Here's the drawing with two shaded views (mm, measured from the low corner). I have some questions. A direction names the side the tool comes from. Give positions to 0.01 mm unless a question says otherwise; leave off trailing zeros. Loops run counter-clockwise (first coordinate to the right, second up) from the corner with the lowest first, then second, coordinate; pieces in that order, holes last. Notation, with made-up numbers: (-12.75, 24.5) -> (-3.75, 24.5) arc R22 cw to (-3.75, 61.5) -> close; hole circle Ø10 at (-13.75, -13). An arc over 180 degrees is marked (long way). Answer in a Markdown table with one row per item. Add a question column.
Item 1: If I drill on line 1 (Y direction, x = 5.75, z = 14.5); line 2 (X direction, y = 59, z = 23); line 3 (Z direction, x = 32, y = 29.5), over which ranges is the centre line in solid material (lowest first)?
Item 2: If we section it at C-C (x = 5.75): Write out the boundary of the cut face in (y, z).
Item 3: If we section it at A-A (z = 11): Write out the boundary of the cut face in (x, y).
Item 4: Which directions (+Z, -Z, +X, -X, +Y, -Y) give clear straight access to the entire face, cutting with the end or side of a thin tool? Please do the marked faces 4, 5 and 6.
Item 5: For P1, Ø16, axis at x = 10, y = 45.5, coming from the -Z side; P2, Ø6.5, axis at x = 5.75, y = 60, coming from the +Z side; P3, Ø10, axis at x = 27, y = 46.5, coming from the -Z side; P4, Ø4.5, axis at x = 31.5, y = 18, coming from the -Z side, each with a flat end and sliding along its axis, tell me the tip position at first contact or that it passes through.
Item 6: If we section it at B-B (y = 10): Write out the boundary of the cut face in (x, z), then the cut area to 3 significant figures.
Item 7: We'd pull the mould along Z, two halves only. Please class the marked faces 1, 2 and 3: released by +Z, released by -Z, zero draft, split by the parting line, or undercut.
Item 8: If we section it at D-D (y = 63): Write out the boundary of the cut face in (x, z), then the cut area to 3 significant figures.
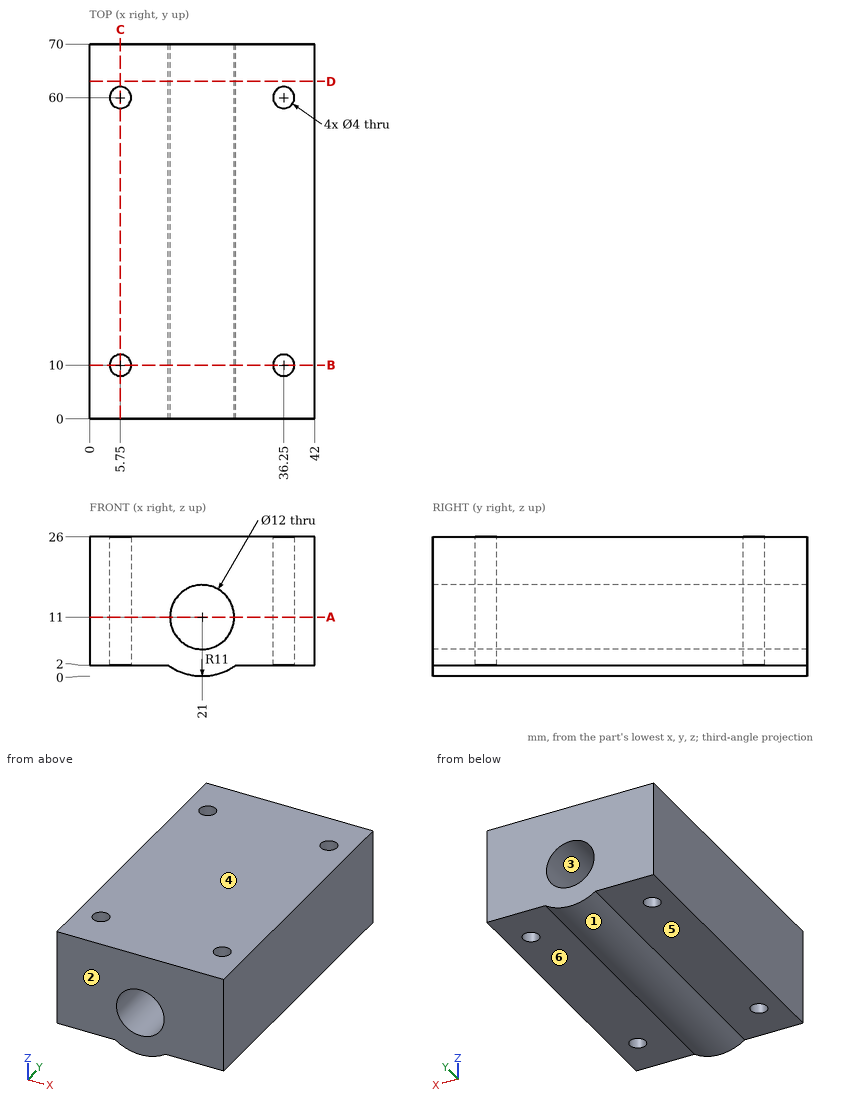
Recorded:
| question | item | result |
|---|---|---|
| 1 | line 1 | y = 0 to 8, 12 to 58, 62 to 70 |
| 1 | line 2 | x = 0 to 4.02, 7.48 to 34.52, 37.98 to 42 |
| 1 | line 3 | z = 2 to 26 |
| 2 | outline | (0, 2) -> (8, 2) -> (8, 26) -> (0, 26) -> close; (12, 2) -> (58, 2) -> (58, 26) -> (12, 26) -> close; (62, 2) -> (70, 2) -> (70, 26) -> (62, 26) -> close |
| 3 | outline | (0, 0) -> (15, 0) -> (15, 70) -> (0, 70) -> close; (27, 0) -> (42, 0) -> (42, 70) -> (27, 70) -> close; hole circle Ø4 at (5.75, 10); hole circle Ø4 at (5.75, 60); hole circle Ø4 at (36.25, 10); hole circle Ø4 at (36.25, 60) |
| 4 | face 4 | +Z, +X, -X, +Y, -Y |
| 4 | face 5 | -Z, -X, +Y, -Y |
| 4 | face 6 | -Z, +X, +Y, -Y |
| 5 | P1 | stops at z = 0.42 |
| 5 | P2 | stops at z = 26 |
| 5 | P3 | stops at z = 0.05 |
| 5 | P4 | stops at z = 2 |
| 6 | outline | (0, 2) -> (3.75, 2) -> (3.75, 26) -> (0, 26) -> close; (7.75, 2) -> (14.68, 2) arc R11 ccw to (27.32, 2) -> (34.25, 2) -> (34.25, 26) -> (7.75, 26) -> close; (38.25, 2) -> (42, 2) -> (42, 26) -> (38.25, 26) -> close; hole circle Ø12 at (21, 11) |
| 6 | area | 720 mm^2 |
| 7 | face 1 | released by -Z |
| 7 | face 2 | zero draft |
| 7 | face 3 | undercut |
| 8 | outline | (0, 2) -> (14.68, 2) arc R11 ccw to (27.32, 2) -> (42, 2) -> (42, 26) -> (0, 26) -> close; hole circle Ø12 at (21, 11) |
| 8 | area | 912 mm^2 |
